from build123d import *

# Parameters (mm, degrees)
F0_W     = 76.2000009418
F0_H     = 45.3736372292
F1_DEPTH = 76.2
F3_DEPTH = 76.201
F4_R     = 7.496665322
F5_DEPTH = 55.7640015627
F6_W     = 94.2109096795
F6_H     = 59.4590939581
F7_DEPTH = 25.4
F9_DEPTH = 101.601


with BuildPart() as f1:
    # F0 (on Front) → F1 (new body)
    with BuildSketch(Plane.XZ):
        with Locations((-38.1000004709, 22.6868186146)):
            Rectangle(F0_W, F0_H)
    extrude(amount=F1_DEPTH)

    # F2 (on face) → F3 (cut, through all)
    with BuildSketch(Plane.XZ.offset(76.2)):
        Polygon((0, 45.3736372292), (-42.2563627362, 45.3736372292), (0, 0), align=None)
    extrude(amount=-F3_DEPTH, mode=Mode.SUBTRACT)

    # F4 (on face) → F5 (cut, through all)
    with BuildSketch(Plane(origin=(0, 0, 0), x_dir=(0, 1, 0), z_dir=(0.7317979117, 0, 0.6815216918))):
        with Locations((-37.869092077, 32.6580442488)):
            Circle(F4_R)
    extrude(amount=-F5_DEPTH, mode=Mode.SUBTRACT)

    # F6 (on face) → F7 (join)
    with BuildSketch(Plane(origin=(0, 0, 0), x_dir=(-1, 0, 0), z_dir=(0, 1, 0))):
        with Locations((29.094546102, 29.7295469791)):
            Rectangle(F6_W, F6_H)
    extrude(amount=F7_DEPTH)

    # F8 (on face) → F9 (cut, through all)
    with BuildSketch(Plane(origin=(0, 25.4, 0), x_dir=(-1, 0, 0), z_dir=(0, 1, 0))):
        Polygon((-18.0109087378, 59.4590939581), (-18.0109087378, 0), (33.2966521382, 59.4590939581), align=None)
    extrude(amount=-F9_DEPTH, mode=Mode.SUBTRACT)


solid = f1.part
The model under review builds one solid part; all positions refer to its coordinate system, in mm. A direction names the side the tool comes from. Coordinates: 2 decimals unless noted, no trailing zeros. Loops run counter-clockwise (first coordinate to the right, second up) from the corner with the lowest first, then second, coordinate; pieces in that order, holes last.
(1) Insertion check: P1, Ø5, axis at y = -50.5, z = 9.5, coming from the +X side; P2, Ø17, axis at x = -56.5, y = -53, coming from the +Z side; P3, Ø1.5, axis at y = 10, z = 50, coming from the +X side. Each pin has a flat end and moves straight along its axis. Give the tip position at first contact, or say it passes through.
Determined:
P1: stops at x = -6.52
P2: stops at z = 45.37
P3: stops at x = -24.49
(2) Consider section D-D, the plane y = -62. Give the boundary of the cut face in (x, z).
Determined:
outline: (-76.2, 0) - (0, 0) - (-42.26, 45.37) - (-76.2, 45.37) - close
(3) Consider section B-B, the plane z = 38. Give the boundary of the cut face in (x, y).
Determined:
outline: (-76.2, -76.2) - (-35.39, -76.2) - (-35.39, 0) - (-14.78, 0) - (-14.78, 25.4) - (-76.2, 25.4) - close
(4) Wall thickness on L1, parallel to Z at x = -64.5, y = -46.5; L2, parallel to Y at x = -44, z = 50; L3, parallel to Z at x = -18, y = 3.5: over which ranges is each line inside the solid? List them lowest first.
Determined:
L1: z = 0 to 45.37
L2: y = 0 to 25.4
L3: z = 0 to 41.73
(5) Consider section C-C, the plane x = -67. Give the boundary of the cut face in (y, z).
Determined:
outline: (-76.2, 0) - (25.4, 0) - (25.4, 59.46) - (0, 59.46) - (0, 45.37) - (-76.2, 45.37) - close
(6) Consider section A-A, the plane y = 3.5. Give the boundary of the cut face in (x, z), plus the area to 3 significant figures.
Determined:
outline: (-76.2, 0) - (18.01, 0) - (-33.3, 59.46) - (-76.2, 59.46) - close
area: 4,080 mm2
(7) Tool access review of faces 4 (the flat face through (-59, -38, 45.374)), 5 (the flat face through (-39, 25.4, 24)), 6 (the flat face through (-16.729, -38.633, 17.963)): name each direction out of +Z, -Z, +X, -X, +Y, -Y from which nothing blocks a thin tool from reaching the whole face with its end or side.
Determined:
face 4: +Z, +X, -X, -Y
face 5: +Z, -Z, +X, -X, +Y
face 6: +Z, +X, -Y
(8) Draft analysis for pull direction Z (two halves, no side actions). For faces 1 (the flat face through (-47, -76.2, 18)), 2 (the cylindrical face through (-39.4, -38.8, 18.1)), 3 (the flat face through (-7.28, 12.88, 29.31)), state which applies: +Z half, -Z half, draft (parallel to the pull), parting line (faces both ways), or undercut.
Determined:
face 1: draft
face 2: undercut
face 3: +Z half
